```python
from build123d import *

# Parameters (mm, degrees)
F1_DEPTH = 3.175
F2_R     = 3.175
F3_DEPTH = 6.351
F4_R     = 3.17499
F5_R     = 3.17499


# Not quite as in the source:
# - a fillet or chamfer is up to 0.001 mm smaller than in the source, because OpenCascade refuses the exact size


with BuildPart() as f1:
    # F0 (on Top) → F1 (new body, symmetric)
    with BuildSketch(Plane.XY):
        with BuildLine():
            Line((101.6, -9.525), (101.6, 9.525))
            Line((101.6, 9.525), (-101.6, 9.525))
            ThreePointArc((-101.6, 9.525), (-111.125, 0), (-101.6, -9.525))
            Line((-101.6, -9.525), (101.6, -9.525))
        make_face()
    extrude(amount=F1_DEPTH, both=True)

    # F2 (on face) → F3 (cut, through all)
    with BuildSketch(Plane.XY.offset(3.175)):
        with Locations((-101.6, 0)):
            Circle(F2_R)
    extrude(amount=-F3_DEPTH, mode=Mode.SUBTRACT)

    # F4 (radius 3.175 in the source; OpenCascade refuses exactly that, so slightly less here)
    f4_edges = [f1.edges().sort_by_distance(p)[0] for p in [
        (0, -9.525, 3.175),
        (-104.775, 0, 3.175),
    ]]
    fillet(f4_edges, radius=F4_R)

    # F5 (radius 3.175 in the source; OpenCascade refuses exactly that, so slightly less here)
    f5_edges = [f1.edges().sort_by_distance(p)[0] for p in [
        (0, -9.525, -3.175),
        (-104.775, 0, -3.175),
    ]]
    fillet(f5_edges, radius=F5_R)


solid = f1.part
```
For this review, take the finished solid that the model builds, in its own axes (mm). Coordinates: 2 decimals unless noted, no trailing zeros. Loops run counter-clockwise (first coordinate to the right, second up) from the corner with the lowest first, then second, coordinate; pieces in that order, holes last. Notation, with made-up numbers: (12, 65) -> (17, 65) arc R27 cw to (17, 91) -> close; hole circle Ø8 at (-15, 32.5). An arc over 180 degrees is marked (long way). Return JSON: item names as keys, results as strings. Group by question number.
(1) For pin 1 Ø10 at (x, y) = (-101.6, 0) entering from -Z; pin 2 Ø1 at (x, z) = (-70, -2) entering from +Y, all flat-tipped, find the tip position at first contact; note any pin that passes through.
(2) Consider section C-C, the plane z = -1.5. Give the boundary of the cut face in (x, y).
(3) To check wall thickness, follow L1, parallel to Y at x = -101.6, z = 0 (3 decimals); L2, parallel to X at y = 0, z = 0.05; L3, parallel to Y at x = 42, z = 0.5. State the ranges of each line that lie inside material, in increasing order.
Results below:
{
 "1": {"pin 1": "stops at z = -2.87", "pin 2": "stops at y = 9.15"},
 "2": {"outline": "(-101.6, -9.15) -> (101.6, -9.15) -> (101.6, 9.15) -> (-101.6, 9.15) arc R9.15 ccw to start; hole circle Ø7.1 at (-101.6, 0)"},
 "3": {"L1": "y = -9.525 to -3.175, 3.175 to 9.525", "L2": "x = -111.12 to -104.78, -98.42 to 101.6", "L3": "y = -9.49 to 9.49"}
}
